from build123d import *

# Parameters (mm, degrees)
SKETCH1_W               = 28.575
SKETCH1_H               = 6.35
EXTRUDE1_DEPTH          = 50.8
EXTRUDE1_DEPTH_BACK     = 50.8
F_1_2_CLEARANCE_HOLE1_D = 13.49248


with BuildPart() as part:
    # Sketch1 → Extrude1 (new body, two sides)
    with BuildSketch(Plane(origin=(0, 0, 0), x_dir=(0, 0, -1), z_dir=(1, 0, 0))) as extrude1_sk:
        Rectangle(SKETCH1_W, SKETCH1_H)
    extrude(amount=EXTRUDE1_DEPTH)
    extrude(extrude1_sk.sketch, amount=-EXTRUDE1_DEPTH_BACK)

    # 1_2 Clearance Hole1 (through all)
    with Locations(Plane(origin=(0, 3.175, 0), x_dir=(-1, 0, 0), z_dir=(0, 1, 0))):
        with Locations((15.875, 0), (-15.875, 0)):
            Hole(F_1_2_CLEARANCE_HOLE1_D / 2)


solid = part.part
The listing builds one solid part. Answer for the finished solid, in the listing's coordinates (mm). Give positions to 0.01 mm unless a question says otherwise; leave off trailing zeros. Write each loop counter-clockwise with the first axis right and the second up, starting at its lowest first coordinate (ties: lowest second). Pieces come first, ordered by that corner, then holes.
1) For a pull along X with two mould halves and no side action, classify faces 1 (the face through (-50.8, 0, 0)), 2 (the face through (9.135, -0.044, 0.297)), 3 (the face through (1, 0, 14.288)), 4 (the face through (-20.847, -0.044, 4.559)) as pulls with the +X half, pulls with the -X half, needs draft (parallel to the pull), parting line crosses it, or undercut.
2) Section B-B (y = 2.25) is taken. Write down the section's boundary in (x, z) (1 decimal), and give its area (3 significant figures).
3) Find the intervals of material crossed by L1, parallel to X at y = -1.5, z = -0.5; L2, parallel to X at y = 0.5, z = 1.75; L3, parallel to Z at x = -10, y = 2.25, in increasing order.
4) Section C-C (x = -13.5) is taken. Write down the section's boundary in (y, z) (1 decimal), and give its area (3 significant figures).
5) Given P1, Ø12, axis at x = -15.875, z = 0, coming from the -Y side, flat-ended and moving along its own axis, determine where the tip first touches the part or whether it passes through.
6) Section A-A (z = 0) is taken. Write down the section's boundary in (x, y) (3 decimals).
Response:
1. face 1: pulls with the -X half
1. face 2: undercut
1. face 3: needs draft
1. face 4: undercut
2. outline: (-50.8, -14.3) - (50.8, -14.3) - (50.8, 14.3) - (-50.8, 14.3) - close; hole circle Ø13.5 at (-15.9, 0); hole circle Ø13.5 at (15.9, 0)
2. area: 2,620 mm2
3. L1: x = -50.8 to -22.6, -9.15 to 9.15, 22.6 to 50.8
3. L2: x = -50.8 to -22.39, -9.36 to 9.36, 22.39 to 50.8
3. L3: z = -14.29 to -3.32, 3.32 to 14.29
4. outline: (-3.2, -14.3) - (3.2, -14.3) - (3.2, -6.3) - (-3.2, -6.3) - close; (-3.2, 6.3) - (3.2, 6.3) - (3.2, 14.3) - (-3.2, 14.3) - close
4. area: 101 mm2
5. P1: passes through
6. outline: (-50.8, -3.175) - (-22.621, -3.175) - (-22.621, 3.175) - (-50.8, 3.175) - close; (-9.129, -3.175) - (9.129, -3.175) - (9.129, 3.175) - (-9.129, 3.175) - close; (22.621, -3.175) - (50.8, -3.175) - (50.8, 3.175) - (22.621, 3.175) - close
